The model under review builds one solid part; all positions refer to its coordinate system, in mm. A direction names the side the tool comes from. Give positions to 0.01 mm unless a question says otherwise; leave off trailing zeros. Order: outer loops, then holes, each group sorted by start corner. A loop starts at its lowest first (then second) coordinate and runs counter-clockwise, first axis right, second up.
```python
from build123d import *

# Parameters (mm, degrees)
F0_R     = 7.5
F1_DEPTH = 3
F2_R     = 0.6
F3_R     = 4
F4_DEPTH = 2


with BuildPart() as f1:
    # F0 (on Front) → F1 (new body)
    with BuildSketch(Plane.XZ):
        Circle(F0_R)
    extrude(amount=F1_DEPTH)

    # F2
    f2_edges = [f1.edges().sort_by_distance(p)[0] for p in [
        (-7.5, -3, 0),
    ]]
    fillet(f2_edges, radius=F2_R)

    # F3 (on face) → F4 (cut)
    with BuildSketch(Plane(origin=(0, 0, 0), x_dir=(-1, 0, 0), z_dir=(0, 1, 0))):
        Circle(F3_R)
    extrude(amount=-F4_DEPTH, mode=Mode.SUBTRACT)


solid = f1.part
```
Item 1: Take a section at A-A (z = 0). Give the boundary of the cut face in (x, y).
Values found:
outline: (-7.5, -2.4) arc R0.6 ccw to (-6.9, -3) - (6.9, -3) arc R0.6 ccw to (7.5, -2.4) - (7.5, 0) - (4, 0) - (4, -2) - (-4, -2) - (-4, 0) - (-7.5, 0) - close
Item 2: Draft analysis for pull direction X (two halves, no side actions). For faces 1 (the flat face through (0, -2, 0)), 2 (the flat face through (0, -3, 0)), 3 (the cylindrical face through (-7.493, -1.183, 0.33)), state which applies: released by +X, released by -X, zero draft, split by the parting line, or undercut.
Values found:
face 1: undercut
face 2: zero draft
face 3: split by the parting line
Item 3: Clearance check with flat-ended pins moving along their axes: pin 1 Ø1.5 at (y, z) = (-2, -2) entering from -X; pin 2 Ø2.5 at (x, z) = (1, -0.5) entering from +Y. State where each tip first meets the part, or that it passes through.
Values found:
pin 1: stops at x = -7.4
pin 2: stops at y = -2
Item 4: Take a section at B-B (y = -1.8). Give the boundary of the cut face in (x, z), and give its area (3 significant figures).
Values found:
outline: circle Ø15 at (0, 0); hole circle Ø8 at (0, 0)
area: 126 mm2
Item 5: For faces 4 (the flat face through (3, 0, -3)), 5 (the cylindrical face through (0.867, -0.986, -3.905)), list the 3-axis set-ups (+Z, -Z, +X, -X, +Y, -Y) from which the entire face can be reached by the end or side of a thin tool; tool diameter is ignored.
Values found:
face 4: +Z, -Z, +X, -X, +Y
face 5: +Y
Item 6: Take a section at C-C (x = 0). Give the boundary of the cut face in (y, z), and give its area (3 significant figures).
Values found:
outline: (-3, -6.9) arc R0.6 ccw to (-2.4, -7.5) - (0, -7.5) - (0, -4) - (-2, -4) - (-2, 4) - (0, 4) - (0, 7.5) - (-2.4, 7.5) arc R0.6 ccw to (-3, 6.9) - close
area: 28.8 mm2
Item 7: For line 1 (Z direction, x = 0, y = -0.75); line 2 (Z direction, x = -3.5, y = -1.95); line 3 (Y direction, x = -2, z = -2.75), list the stretches that pass through material, from the lowest coordinate up.
Values found:
line 1: z = -7.5 to -4, 4 to 7.5
line 2: z = -6.63 to -1.94, 1.94 to 6.63
line 3: y = -3 to -2
